Autodesk Inventor part; units mm, degrees
ref_plane "YZ Plane" through (0, 0, 0) normal (1, 0, 0) x (0, 1, 0)
ref_plane "XZ Plane" through (0, 0, 0) normal (0, 1, 0) x (-1, 0, 0)
ref_plane "XY Plane" through (0, 0, 0) normal (0, 0, 1) x (1, 0, 0)
sketch "Sketch1" plane through (0, 0, 0) normal (0, 0, 1) x (1, 0, 0)
  line L0 (-15, 0) -> (-6.35, 0)
  line L1 (-6.35, 0) -> (-6.35, 15)
  line L2 (-6.35, 15) -> (-7.5, 15)
  line L3 (-7.5, 15) -> (-7.5, 3)
  line L4 (-7.5, 3) -> (-15, 3)
  line L5 (-15, 3) -> (-15, 0)
  line L6 (0, -3) -> (0, 18)
  point P0 (0, 0)
  dimension "d0" = 3
  dimension "d2" = 15
  dimension "d3" = 6.35
  dimension "d4" = 15
  dimension "d17" = 7.5
  dimension "d18" = 1.15
revolve "Revolution1" add sketch "Sketch1" angle 360 about axis through (0, -10, 0) along (0, 1, 0)
sketch "Sketch2" plane through (0, 3, 0) normal (0, 1, 0) x (1, 0, 0)
  point P0 (0, 0)
  point P1 (0.0472, 12)
  point P2 (0, -12)
  dimension "d6" = 12
  dimension "d22" = 12
hole "Hole1" at (0.0472, 3, -12) at (0, 3, 12) direction (0, -1, 0) diameter 2.459 end through all
sketch "Sketch4" plane through (0, 3, 0) normal (0, 1, 0) x (1, 0, 0)
  circle A0 centre (0, 0) radius 15
  circle A1 centre (0, 0) radius 7.5
  circle A2 centre (-55, 0) radius 64
  point P0 (7.6909, 12.8783)
  point P1 (7.5, 0)
  point P2 (7.6909, -12.8783)
  dimension "d23" = 128
  dimension "d24" = 55
extrude "Extrusion2" cut sketch "Sketch4" against normal through all contours A0 A2 picked at (10.8452, -2.4648)
sketch "Sketch6" plane through (0, 3, 0) normal (0, 1, 0) x (1, 0, 0)
  arc A0 (7.6909, 12.8783) -> (7.6909, -12.8783) centre (0, 0) ccw
  circle A1 centre (0, 0) radius 7.5
  line L0 (-6.3443, 4) -> (-15, 4)
  line L1 (-15, 4) -> (-15, -4)
  line L2 (-15, -4) -> (-6.3443, -4)
  line L3 (-6.3443, -4) -> (-6.3443, 4)
  point P0 (-14.4568, -4)
  point P1 (-6.3443, -4)
  point P2 (-14.4568, 4)
  dimension "d32" = 4
  dimension "d33" = 4
extrude "Extrusion3" add sketch "Sketch6" along normal up to surface (12 mm away) contours L0 A1 L2 A0
sketch "Sketch7" plane through (-14.4568, 15, -4) normal (0, 1, 0) x (1, 0, 0)
  circle A0 centre (14.4568, -4) radius 6.35
  line L0 (8.1861, -5) -> (-0.5432, -5)
  line L1 (-0.5432, -5) -> (-0.5432, -3)
  line L2 (-0.5432, -3) -> (8.1861, -3)
  line L3 (8.1861, -3) -> (8.1861, -5)
  arc A1 (0, 0) -> (0, -8) centre (14.4568, -4) ccw
  point P0 (-0.5098, -5)
  point P1 (8.1861, -3)
  point P2 (-0.5098, -3)
  dimension "d27" = 1
  dimension "d28" = 1
extrude "Extrusion4" cut sketch "Sketch7" against normal through all contours A0 L0 A1 L2
sketch "Sketch8" plane through (-14.4568, 3, 4) normal (0, 0, 1) x (1, 0, 0)
  line L0 (0, 0) -> (0, 12)
  line L1 (8.1125, 12) -> (0, 12)
  point P0 (7.0914, 12)
  point P1 (4, 6)
  dimension "d35" = 12
  dimension "d37" = 4
  dimension "d38" = 6
hole "Hole2" at (-10.4568, 9, 4) direction (0, 0, -1) diameter 4 end through all
properties part number "BaffleClampWithScrew" material "Brass, Soft Yellow"
Input: part model. Units: mm. Frame: model coordinates. A direction names the side the tool comes from. Round coordinates to 2 decimals unless told otherwise and drop trailing zeros. Loops run counter-clockwise (first coordinate to the right, second up) from the corner with the lowest first, then second, coordinate; pieces in that order, holes last. Notation, with made-up numbers: (72, 86.25) -> (127, 86.25) arc R17 cw to (127, 110.25) -> close; hole circle Ø3 at (-25, 69.25). An arc over 180 degrees is marked (long way). One line per item, written item: value.
(1) Material intervals for line 1 (Z direction, x = 0, y = 1.65); line 2 (Z direction, x = -8, y = 7.75); line 3 (X direction, y = 9, z = -1.8), sorted ascending. Write a range as [from, to].
Geometry check:
line 1: [-15, -13.23], [-10.77, -6.35], [6.35, 10.77], [13.23, 15]
line 2: [-4, -1], [1, 4]
line 3: [-14.89, -12.46], [-8.46, -6.09], [6.09, 7.28]
(2) Pin query (flat end, axial travel): pin 1 (6.5 mm diameter, centred on x = -10.46, y = 9, fed in from -Z); pin 2 (1 mm diameter, centred on y = 6.5, z = 6, fed in from -X); pin 3 (3 mm diameter, centred on x = 0, z = 9.5, fed in from +Y); pin 4 (2.5 mm diameter, centred on x = -10.5, y = 9.5, fed in from +Z). Return the tip coordinate at first contact, or that it passes through.
Geometry check:
pin 1: z = -4
pin 2: x = -5.1
pin 3: y = 3
pin 4: through
(3) Mould query, pull axis Y, two halves, no side actions, for faces 1 (the face through (-8.5, 10.2, -4)), 2 (the face through (-5, 3, 7)), 3 (the face through (-8.68, 8.08, -2.52)). Classes: pulls with the +Y half, pulls with the -Y half, needs draft (parallel to the pull), parting line crosses it, or undercut.
Geometry check:
face 1: needs draft
face 2: pulls with the +Y half
face 3: undercut
(4) Section B-B (z = 2.5). Return the cut outline in (x, y).
Geometry check:
outline: (-14.79, 0) -> (-5.84, 0) -> (-5.84, 15) -> (-14.79, 15) -> close; (5.84, 0) -> (8.95, 0) -> (8.95, 3) -> (7.07, 3) -> (7.07, 15) -> (5.84, 15) -> close; hole circle Ø4 at (-10.46, 9)
(5) Section D-D (y = 4.25). Return the cut outline in (x, z).
Geometry check:
outline: (-14.97, -1) arc R15 ccw to (-14.46, -4) -> (-6.34, -4) arc R7.5 ccw (long way) to (-6.34, 4) -> (-14.46, 4) arc R15 ccw to (-14.97, 1) -> (-6.27, 1) arc R6.35 cw (long way) to (-6.27, -1) -> close
(6) Section A-A (y = 9). Return the cut outline in (x, z).
Geometry check:
outline: (-14.97, -1) arc R15 ccw to (-14.46, -4) -> (-12.46, -4) -> (-12.46, -1) -> close; (-14.97, 1) -> (-12.46, 1) -> (-12.46, 4) -> (-14.46, 4) arc R15 ccw to start; (-8.46, -4) -> (-6.34, -4) arc R7.5 ccw (long way) to (-6.34, 4) -> (-8.46, 4) -> (-8.46, 1) -> (-6.27, 1) arc R6.35 cw (long way) to (-6.27, -1) -> (-8.46, -1) -> close
(7) Set-up query: faces 4 (the face through (-8.65, 10.25, 4)), 5 (the face through (7.495, 8.916, -0.271)), 6 (the face through (-11, 6, -1)). Return all of +Z, -Z, +X, -X, +Y, -Y with unobstructed straight access to the full face (end or side cutting, diameter ignored); none if empty.
Geometry check:
face 4: +Z, -X, +Y
face 5: +Y
face 6: -X, +Y, -Y
(8) Section C-C (x = -1.75). Return the cut outline in (y, z).
Geometry check:
outline: (0, -14.9) -> (3, -14.9) -> (3, -7.29) -> (15, -7.29) -> (15, -6.1) -> (0, -6.1) -> close; (0, 6.1) -> (15, 6.1) -> (15, 7.29) -> (3, 7.29) -> (3, 14.9) -> (0, 14.9) -> close
